The listing builds one solid part. Answer for the finished solid, in the listing's coordinates (mm). A direction names the side the tool comes from. Give positions to 0.01 mm unless a question says otherwise; leave off trailing zeros. Loops run counter-clockwise (first coordinate to the right, second up) from the corner with the lowest first, then second, coordinate; pieces in that order, holes last. Notation, with made-up numbers: (-29.75, -29.5) - (6.25, -29.5) arc R22 cw to (6.25, 4.5) - close; hole circle Ø11 at (78.5, 61). An arc over 180 degrees is marked (long way). Write each question's results on one line, items separated by ' | '.
from build123d import *

# Parameters (mm, degrees)
SKETCH1_W                    = 80
SKETCH1_H                    = 12.7
BOSS_EXTRUDE1_DEPTH          = 3.175
EDGE_FLANGE1_STRIP_W         = 14.7
EDGE_FLANGE1_STRIP_H         = 3.175
EDGE_FLANGE1_STRIP_CUT_DEPTH = 12.7
EDGE_FLANGE1_DEPTH           = 12.7
EDGE_FLANGE2_STRIP_W         = 14.7
EDGE_FLANGE2_STRIP_H         = 3.175
EDGE_FLANGE2_STRIP_CUT_DEPTH = 12.7
EDGE_FLANGE2_DEPTH           = 12.7
M8_CLEARANCE_HOLE1_D         = 9


# Sheet-metal steps are written as plain solids
with BuildPart() as part:
    # Sketch1 → Boss-Extrude1 (new body)
    with BuildSketch(Plane(origin=(0, 0, 0), x_dir=(1, 0, 0), z_dir=(0, 1, 0))):
        with Locations((40, 6.35)):
            Rectangle(SKETCH1_W, SKETCH1_H)
    extrude(amount=BOSS_EXTRUDE1_DEPTH)

    # Edge-Flange1 strip (across the edge) → Edge-Flange1 strip cut (cut)
    with BuildSketch(Plane(origin=(80, 3.175, 0), x_dir=(-1, 0, 0), z_dir=(0, 0, -1))):
        with Locations((-3.175, -1.5875)):
            Rectangle(EDGE_FLANGE1_STRIP_W, EDGE_FLANGE1_STRIP_H)
    extrude(amount=EDGE_FLANGE1_STRIP_CUT_DEPTH, mode=Mode.SUBTRACT)

    # Edge-Flange1 section (across the edge) → Edge-Flange1 (add)
    with BuildSketch(Plane(origin=(80, 3.175, 0), x_dir=(-1, 0, 0), z_dir=(0, 0, -1))):
        with BuildLine():
            Line((0, 1), (0, 41.32))
            Line((0, 41.32), (3.175, 41.32))
            Line((3.175, 41.32), (3.175, 1))
            ThreePointArc((3.175, 1), (3.467893219, 0.292893219), (4.175, 0))
            Line((4.175, 0), (4.175, -3.175))
            ThreePointArc((4.175, -3.175), (1.222829189, -1.952170811), (0, 1))
        make_face()
    extrude(amount=EDGE_FLANGE1_DEPTH)

    # Edge-Flange2 strip (across the edge) → Edge-Flange2 strip cut (cut)
    with BuildSketch(Plane(origin=(80, 44.495, -12.7), x_dir=(0, -1, 0), z_dir=(0, 0, 1))):
        with Locations((-3.175, -1.5875)):
            Rectangle(EDGE_FLANGE2_STRIP_W, EDGE_FLANGE2_STRIP_H)
    extrude(amount=EDGE_FLANGE2_STRIP_CUT_DEPTH, mode=Mode.SUBTRACT)

    # Edge-Flange2 section (across the edge) → Edge-Flange2 (add)
    with BuildSketch(Plane(origin=(80, 44.495, -12.7), x_dir=(0, -1, 0), z_dir=(0, 0, 1))):
        with BuildLine():
            Line((0, 1), (0, 41.825))
            Line((0, 41.825), (3.175, 41.825))
            Line((3.175, 41.825), (3.175, 1))
            ThreePointArc((3.175, 1), (3.467893219, 0.292893219), (4.175, 0))
            Line((4.175, 0), (4.175, -3.175))
            ThreePointArc((4.175, -3.175), (1.222829189, -1.952170811), (0, 1))
        make_face()
    extrude(amount=EDGE_FLANGE2_DEPTH)

    # M8 Clearance Hole1 (through all)
    with Locations(Plane(origin=(0, 44.495, 0), x_dir=(1, 0, 0), z_dir=(0, 1, 0))):
        with Locations((111.825, 6.35), (10, 6.35)):
            Hole(M8_CLEARANCE_HOLE1_D / 2)


solid = part.part
Item 1: A cutting plane is placed at D-D, the plane x = 65.5. Determine the outline of the cut face in (y, z) (3 decimals).
Values found:
outline: (0, -12.7) - (3.175, -12.7) - (3.175, 0) - (0, 0) - close
Item 2: For faces 5 (the face through (102, 41.32, -6)), 6 (the face through (37, 3.175, -6)), 7 (the face through (0, 2, -6)), determine the directions among +Z, -Z, +X, -X, +Y, -Y from which every point of the face is accessible in a straight line to the end or side of a thin tool.
Values found:
face 5: +Z, -Z, +X, -Y | face 6: +Z, -Z, -X, +Y | face 7: +Z, -Z, -X, +Y, -Y
Item 3: A cutting plane is placed at B-B, the plane x = 10. Determine the outline of the cut face in (y, z) (3 decimals).
Values found:
outline: (0, -12.7) - (3.175, -12.7) - (3.175, -10.85) - (0, -10.85) - close; (0, -1.85) - (3.175, -1.85) - (3.175, 0) - (0, 0) - close
Item 4: A cutting plane is placed at C-C, the plane y = 18.5. Determine the outline of the cut face in (x, z) (3 decimals).
Values found:
outline: (76.825, -12.7) - (80, -12.7) - (80, 0) - (76.825, 0) - close
Item 5: A cutting plane is placed at A-A, the plane z = -6.35. Determine the outline of the cut face in (x, y) (3 decimals), plus the area to 3 significant figures.
Values found:
outline: (0, 0) - (5.5, 0) - (5.5, 3.175) - (0, 3.175) - close; (14.5, 0) - (75.825, 0) arc R4.175 ccw to (80, 4.175) - (80, 40.32) arc R1 cw to (81, 41.32) - (107.325, 41.32) - (107.325, 44.495) - (81, 44.495) arc R4.175 ccw to (76.825, 40.32) - (76.825, 4.175) arc R1 cw to (75.825, 3.175) - (14.5, 3.175) - close; (116.325, 41.32) - (121.825, 41.32) - (121.825, 44.495) - (116.325, 44.495) - close | area: 454 mm²
Item 6: For a pull along Z with two mould halves and no side action, classify faces 1 (the face through (79, 19, 0)), 2 (the face through (116.32, 42.89, -6.55)), 3 (the face through (121.825, 43, -6)), 4 (the face through (5.708, 1.565, -7.702)) as released by +Z, released by -Z, zero draft, split by the parting line, or undercut.
Values found:
face 1: released by +Z | face 2: undercut | face 3: zero draft | face 4: undercut
Item 7: Find the intervals of material crossed by line 1 along Z through (x, y) = (10, 1); line 2 along Y through (x, z) = (100, -9.5) (3 decimals); line 3 along Y through (x, z) = (49, -0.75) (3 decimals), in increasing order. Write a range as [from, to].
Values found:
line 1: z = [-12.7, -10.85], [-1.85, 0] | line 2: y = [41.32, 44.495] | line 3: y = [0, 3.175]
Item 8: Flat-ended cylindrical pins translate along their axes: P1, Ø6.5, axis at y = 15.5, z = -7, coming from the +X side; P2, Ø1, axis at x = 83.5, z = -7, coming from the -Y side; P3, Ø2, axis at x = 34.5, z = -8, coming from the +Y side (3 decimals). Find the tip coordinate at first contact, or state that the pin passes through.
Values found:
P1: stops at x = 80 | P2: stops at y = 41.32 | P3: stops at y = 3.175
